Solid Edge part; units mm, degrees
sketch "Sketch1" plane through (0, 0, 0) normal (0, -1, 0) x (1, 0, 0)
  line L0 (-59, -40) -> (-59, 40)
  line L1 (-59, 40) -> (59, 40)
  line L2 (59, 40) -> (59, -40)
  line L3 (59, -40) -> (-59, -40)
extrude "Protrusion1" add sketch "Sketch1" against normal blind 10
extrude "Extrusionsausschnitt_1" [suppressed]
hole "Bohrung_1" at (34, 0, -34) direction (0, 1, 0) diameter 6.6 end up to next
hole "Hole1" at (-34, 0, -34) direction (0, 1, 0) diameter 6.6 end up to next
hole "Hole2" at (-34, 0, 34) direction (0, 1, 0) diameter 6.6 end up to next
hole "Hole3" at (34, 0, 34) direction (0, 1, 0) diameter 6.6 end up to next
hole "Bohrung_5" at (51.5, 10, -20) direction (0, -1, 0) diameter 6.6 end up to next
hole "Hole4" at (-51.5, 10, -20) direction (0, -1, 0) diameter 6.6 end up to next
hole "Hole5" at (-51.5, 10, 20) direction (0, -1, 0) diameter 6.6 end up to next
hole "Hole6" at (51.5, 10, 20) direction (0, -1, 0) diameter 6.6 end up to next
hole "Bohrung_9" at (43, 5, -40) direction (0, 0, 1) diameter 4.917 depth 25 tip angle 118 thread major 6 thread length 20
hole "Hole7" at (-43, 5, -40) direction (0, 0, 1) diameter 4.917 depth 25 tip angle 118 thread major 6 thread length 20
mirror "Mirror1" about plane through (0, 0, 0) normal (0, 0, -1) of "Bohrung_9", "Hole7"
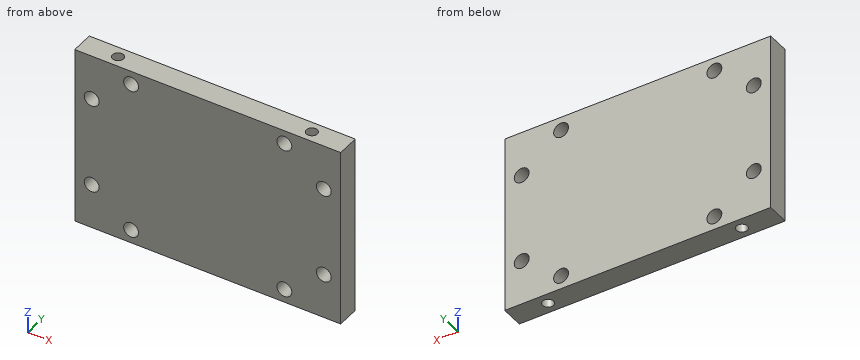
Input: part model. Units: mm. Frame: model coordinates. Give positions to 0.01 mm unless a question says otherwise; leave off trailing zeros. Write each loop counter-clockwise with the first axis right and the second up, starting at its lowest first coordinate (ties: lowest second). Pieces come first, ordered by that corner, then holes. Notation, with made-up numbers: (28, -29.5) - (53, -29.5) arc R36 cw to (53, 8.5) - close; hole circle Ø8 at (52, -32). An arc over 180 degrees is marked (long way). Write item = value, one per line. Start each with the question number.
1) Pin query (flat end, axial travel): pin 1 (1.5 mm diameter, centred on x = 8, z = -27.5, fed in from -Y); pin 2 (4 mm diameter, centred on x = -43, y = 5, fed in from -Z); pin 3 (4.5 mm diameter, centred on x = 43, y = 5, fed in from +Z); pin 4 (3 mm diameter, centred on x = 43, y = 5, fed in from -Z). Return the tip coordinate at first contact, or that it passes through.
2) Material intervals for L1, parallel to Z at x = -34, y = 3.75; L2, parallel to Z at x = 51.5, y = 4.25; L3, parallel to X at y = 7.5, z = -34, sorted ascending. Write a range as [from, to].
3) Cut plane C-C (z = -21.5). Return loops of the section in (x, y), and give its area (3 significant figures).
4) Cut plane B-B (x = -34). Return loops of the section in (y, z).
5) Cut plane A-A (z = -34). Return loops of the section in (x, y).
6) Cut plane D-D (x = 49.5). Return loops of the section in (y, z).
Answers follow:
q1.pin_1 = 0
q1.pin_2 = -14.72
q1.pin_3 = 14.87
q1.pin_4 = -14.42
q2.L1 = [-40, -37.3], [-30.7, 30.7], [37.3, 40]
q2.L2 = [-40, -23.3], [-16.7, 16.7], [23.3, 40]
q2.L3 = [-59, -37.3], [-30.7, 30.7], [37.3, 59]
q3.outline = (-59, 0) - (-54.44, 0) - (-54.44, 10) - (-59, 10) - close; (-48.56, 0) - (48.56, 0) - (48.56, 10) - (-48.56, 10) - close; (54.44, 0) - (59, 0) - (59, 10) - (54.44, 10) - close; hole circle Ø4.92 at (-43, 5); hole circle Ø4.92 at (43, 5)
q3.area = 1,020 mm^2
q4.outline = (0, -40) - (10, -40) - (10, -37.3) - (0, -37.3) - close; (0, -30.7) - (10, -30.7) - (10, 30.7) - (0, 30.7) - close; (0, 37.3) - (10, 37.3) - (10, 40) - (0, 40) - close
q5.outline = (-59, 0) - (-37.3, 0) - (-37.3, 10) - (-59, 10) - close; (-30.7, 0) - (30.7, 0) - (30.7, 10) - (-30.7, 10) - close; (37.3, 0) - (59, 0) - (59, 10) - (37.3, 10) - close; hole circle Ø4.92 at (-43, 5); hole circle Ø4.92 at (43, 5)
q6.outline = (0, -40) - (10, -40) - (10, -22.62) - (0, -22.62) - close; (0, -17.38) - (10, -17.38) - (10, 17.38) - (0, 17.38) - close; (0, 22.62) - (10, 22.62) - (10, 40) - (0, 40) - close
